Could you check a few things on this drawing? It's one solid part, dimensions in mm from its lowest x, y, z. A direction names the side the tool comes from. Give positions to 0.01 mm unless a question says otherwise; leave off trailing zeros. Loops run counter-clockwise (first coordinate to the right, second up) from the corner with the lowest first, then second, coordinate; pieces in that order, holes last. Notation, with made-up numbers: (48.25, 14) - (61.25, 14) arc R18 ccw to (61.25, 34) - close; hole circle Ø5 at (40, 69.5). An arc over 180 degrees is marked (long way). Use a Markdown table: item, result.
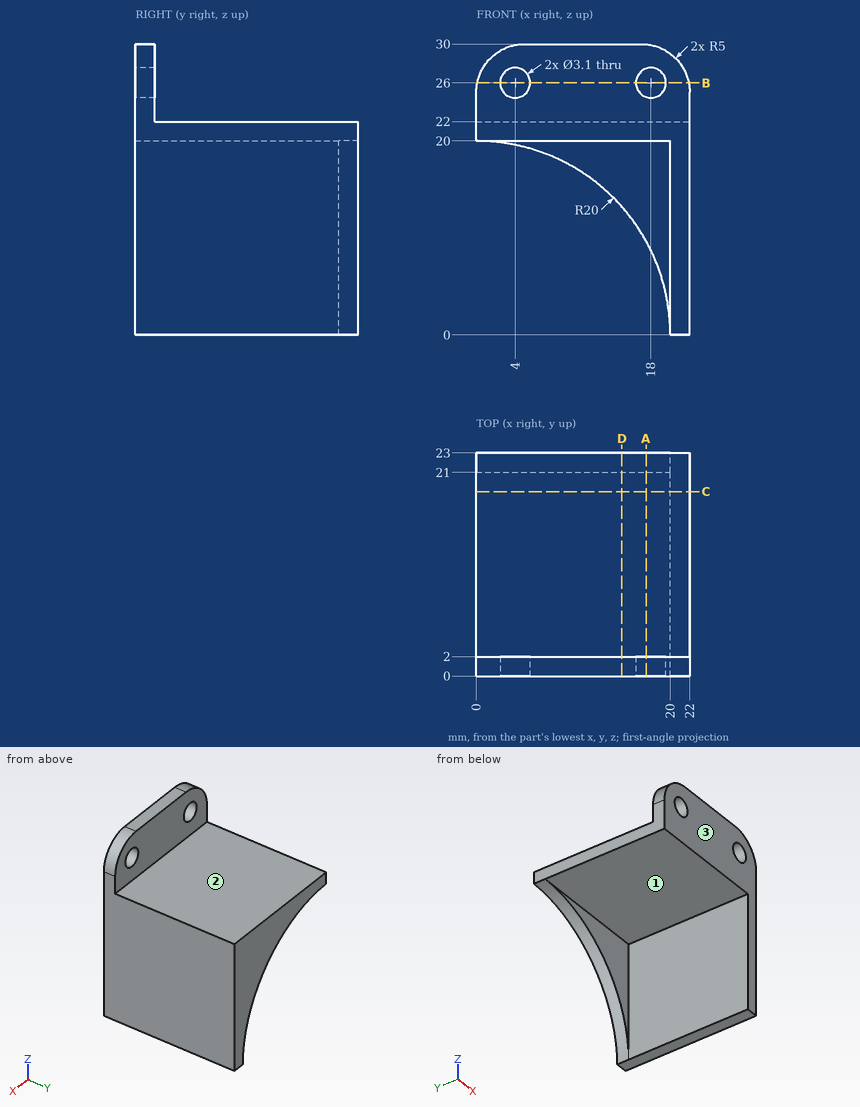
(1) Suppose I cut it at B-B on z = 26. Write out the boundary of the cut face in (x, y).
A:
| item | result |
|---|---|
| outline | (0.1, 0) - (2.45, 0) - (2.45, 2) - (0.1, 2) - close; (5.55, 0) - (16.45, 0) - (16.45, 2) - (5.55, 2) - close; (19.55, 0) - (21.9, 0) - (21.9, 2) - (19.55, 2) - close |
(2) Suppose I cut it at C-C on y = 19. Write out the boundary of the cut face in (x, z), plus the area to 3 significant figures.
A:
| item | result |
|---|---|
| outline | (0, 20) - (20, 20) - (20, 0) - (22, 0) - (22, 22) - (0, 22) - close |
| area | 84.0 mm2 |
(3) Suppose I cut it at D-D on x = 15. Write out the boundary of the cut face in (y, z).
A:
| item | result |
|---|---|
| outline | (0, 20) - (21, 20) - (21, 13.23) - (23, 13.23) - (23, 22) - (2, 22) - (2, 30) - (0, 30) - close |
(4) Will these pins go through, and if not, where does the flat tip stop? pin 1 (2 mm diameter, centred on y = 12.5, z = 17, fed in from -X); pin 2 (5 mm diameter, centred on x = 9, z = 17, fed in from -Y); pin 3 (12 mm diameter, centred on x = 4.5, z = 10.5, fed in from +Y); pin 4 (3 mm diameter, centred on x = 13.5, y = 11, fed in from +Z).
A:
| item | result |
|---|---|
| pin 1 | x = 20 |
| pin 2 | y = 21 |
| pin 3 | through |
| pin 4 | z = 22 |
(5) Suppose I cut it at A-A on x = 17.5. Write out the boundary of the cut face in (y, z), plus the area to 3 significant figures.
A:
| item | result |
|---|---|
| outline | (0, 20) - (21, 20) - (21, 9.68) - (23, 9.68) - (23, 22) - (2, 22) - (2, 24.53) - (0, 24.53) - close; (0, 27.47) - (2, 27.47) - (2, 29.97) - (0, 29.97) - close |
| area | 76.7 mm2 |
(6) If I drill on line 1 (Z direction, x = 9, y = 5.25); line 2 (Y direction, x = 19, z = 14.25); line 3 (Y direction, x = 16, z = 24), over which ranges is the centre line in solid material (lowest first)?
A:
| item | result |
|---|---|
| line 1 | 20 to 22 |
| line 2 | 21 to 23 |
| line 3 | 0 to 2 |
(7) On a 3-axis mill with a long thin cutter (end or side, diameter ignored), from which of +Z, -Z, +X, -X, +Y, -Y can I reach the whole of each face in a straight line? I mean the marked faces 1, 2 and 3. Say none if no direction works.
A:
| item | result |
|---|---|
| face 1 | -Z, -X, -Y |
| face 2 | +Z, +X, -X, +Y |
| face 3 | +Z, -Z, +X, -X, -Y |
